Could you check a few things on this drawing? It's one solid part, dimensions in mm from its lowest x, y, z. Coordinates: 2 decimals unless noted, no trailing zeros. Write each loop counter-clockwise with the first axis right and the second up, starting at its lowest first coordinate (ties: lowest second). Pieces come first, ordered by that corner, then holes. Notation, with made-up numbers: M 26.5,35 L 83.5,35 A10 cw 83.5,39 Z; hole C 21,9.5 d8. An arc over 180 degrees is marked long. Use a Markdown table: item, result.
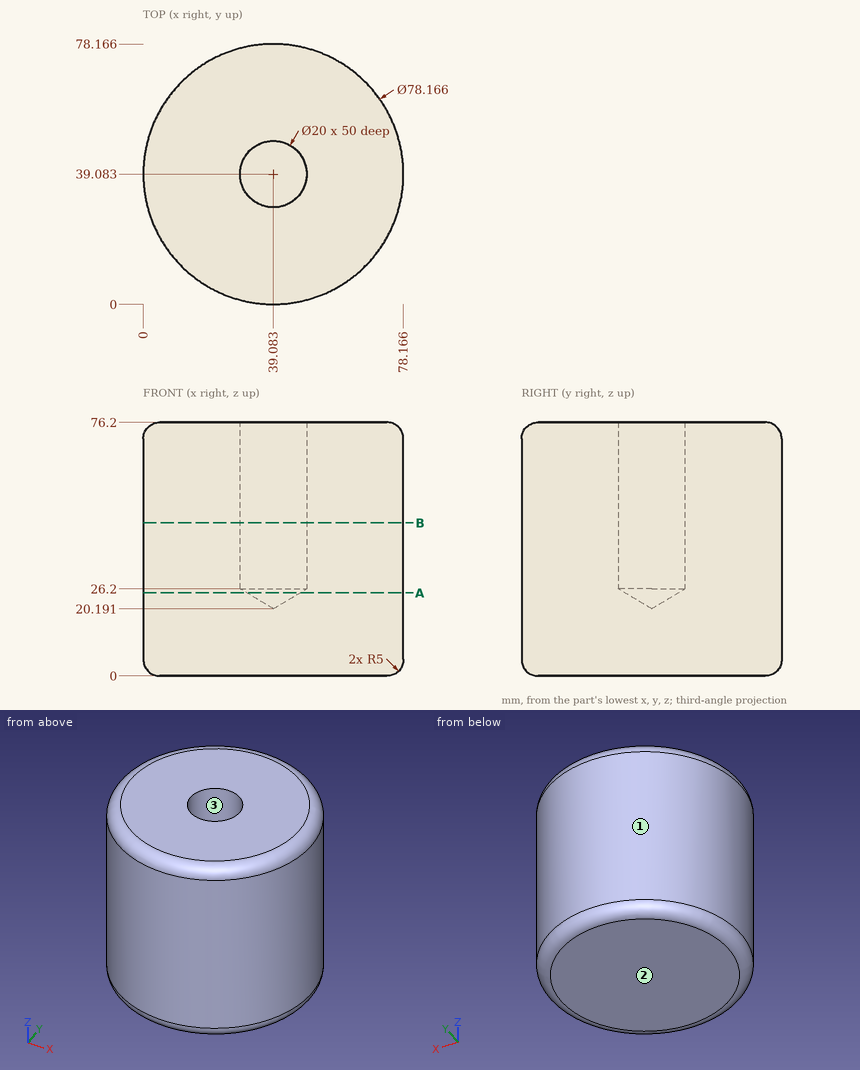
1. I need wall thicknesses on probe 1 along Y at (x, z) = (39.5, 51.5) (1 decimal); probe 2 along X at (y, z) = (35.5, 58) (1 decimal); probe 3 along Y at (x, z) = (47, 26.5) (1 decimal). Which ranges of each line are inside material? Lowest first, please.
Answers follow:
| item | result |
|---|---|
| probe 1 | y = 0 to 29.1, 49.1 to 78.2 |
| probe 2 | x = 0.2 to 29.7, 48.4 to 78 |
| probe 3 | y = 0.8 to 33, 45.2 to 77.4 |
2. We'd pull the mould along Y, two halves only. Please class the marked faces 1, 2 and 3: +Y half, -Y half, draft (parallel to the pull), parting line (faces both ways), or undercut.
Answers follow:
| item | result |
|---|---|
| face 1 | parting line |
| face 2 | draft |
| face 3 | undercut |
3. Suppose I cut it at A-A on z = 25. Write out the boundary of the cut face in (x, y) (1 decimal).
Answers follow:
| item | result |
|---|---|
| outline | C 39.1,39.1 d78.2; hole C 39.1,39.1 d16 |
4. Will these pins go through, and if not, where does the flat tip stop? pin 1 Ø6 at (y, z) = (20, 22.5) entering from -X; pin 2 Ø6 at (y, z) = (33.5, 37.5) entering from -X (1 decimal); pin 3 Ø2 at (y, z) = (48.5, 9.5) entering from -X; pin 4 Ø3 at (x, y) = (22, 40) entering from -Z.
Answers follow:
| item | result |
|---|---|
| pin 1 | stops at x = 3.46 |
| pin 2 | stops at x = 0.1 |
| pin 3 | stops at x = 0.92 |
| pin 4 | stops at z = 0 |
5. Suppose I cut it at B-B on z = 46. Write out the boundary of the cut face in (x, y).
Answers follow:
| item | result |
|---|---|
| outline | C 39.08,39.08 d78.17; hole C 39.08,39.08 d20 |
